from build123d import *

# Parameters (mm, degrees)
F0_W     = 74
F0_H     = 88.5
F1_DEPTH = 34
F2_W     = 70
F2_H     = 83.5
F3_DEPTH = 33
F5_DEPTH = 15
F6_DEPTH = 1
F7_W     = 10
F7_H     = 6
F8_DEPTH = 25


with BuildPart() as f1:
    # F0 (on Top) → F1 (new body)
    with BuildSketch(Plane.XY):
        Rectangle(F0_W, F0_H)
    extrude(amount=F1_DEPTH)

    # F2 (on face) → F3 (cut)
    with BuildSketch(Plane.XY.offset(34)):
        Rectangle(F2_W, F2_H)
    extrude(amount=-F3_DEPTH, mode=Mode.SUBTRACT)

    # F4 (on face) → F5 (join)
    with BuildSketch(Plane.XY.offset(1)):
        with BuildLine():
            ThreePointArc((-7.5, 39.25), (-7.866117, 40.133883), (-8.75, 40.5))
            Line((-8.75, 40.5), (-8.75, 39.25))
            Line((-8.75, 39.25), (-10, 39.25))
            ThreePointArc((-10, 39.25), (-8.75, 38), (-7.5, 39.25))
        make_face()
        with BuildLine():
            Line((-8.75, 39.25), (-8.75, 40.5))
            ThreePointArc((-8.75, 40.5), (-9.633883, 40.133883), (-10, 39.25))
            Line((-10, 39.25), (-8.75, 39.25))
        make_face()
    extrude(amount=F5_DEPTH)

    # F0 (on Top) → F6 (join)
    with BuildSketch(Plane.XY):
        Rectangle(F0_W, F0_H)
    extrude(amount=-F6_DEPTH)

    # F7 (on face) → F8 (cut)
    with BuildSketch(Plane.XZ.offset(44.25)):
        with Locations((-12, 10.5)):
            Rectangle(F7_W, F7_H)
    extrude(amount=-F8_DEPTH, mode=Mode.SUBTRACT)


solid = f1.part
Input: part model. Units: mm. Frame: model coordinates. A direction names the side the tool comes from. Round coordinates to 2 decimals unless told otherwise and drop trailing zeros. Order: outer loops, then holes, each group sorted by start corner. A loop starts at its lowest first (then second) coordinate and runs counter-clockwise, first axis right, second up. Notation, with made-up numbers: (-8, 54) - (49, 54) arc R16 cw to (49, 68) - close; hole circle Ø1 at (2, -35.5). An arc over 180 degrees is marked (long way). Use a Markdown table: item, result.
1. Material intervals for probe 1 along Y at (x, z) = (24.5, 25); probe 2 along X at (y, z) = (-39, 3.5); probe 3 along Y at (x, z) = (-11.5, 12.5), sorted ascending.
Evaluation:
| item | result |
|---|---|
| probe 1 | -44.25 to -41.75, 41.75 to 44.25 |
| probe 2 | -37 to -35, 35 to 37 |
| probe 3 | 41.75 to 44.25 |
2. First-contact query: pin 1 (1.2 mm diameter, centred on x = -9, y = 39, fed in from +Z). Flat tip, straight axial feed; report the tip coordinate or a pass-through.
Evaluation:
| item | result |
|---|---|
| pin 1 | z = 16 |
3. Access query for faces 1 (the face through (0, 1, 1)), 2 (the face through (-12, -43, 7.5)), 3 (the face through (-36, 0, 34)). Directions: +Z, -Z, +X, -X, +Y, -Y. A direction counts if a zero-diameter tool reaches every point of the face in a straight line with its end or side. Return the directions, or none.
Evaluation:
| item | result |
|---|---|
| face 1 | +Z |
| face 2 | -Y |
| face 3 | +Z, +X, -X, +Y, -Y |
4. Section B-B on z = 19. Return the cut outline in (x, y), then the cut area to 3 significant figures.
Evaluation:
| item | result |
|---|---|
| outline | (-37, -44.25) - (37, -44.25) - (37, 44.25) - (-37, 44.25) - close; hole (-35, -41.75) - (35, -41.75) - (35, 41.75) - (-35, 41.75) - close |
| area | 704 mm^2 |
5. Section A-A on z = 3.5. Return the cut outline in (x, y), then the cut area to 3 significant figures.
Evaluation:
| item | result |
|---|---|
| outline | (-37, -44.25) - (37, -44.25) - (37, 44.25) - (-37, 44.25) - close; (-10, 39.25) arc R1.25 ccw to (-7.5, 39.25) arc R1.25 ccw to (-8.75, 40.5) arc R1.25 ccw to start; hole (-35, -41.75) - (35, -41.75) - (35, 41.75) - (-35, 41.75) - close |
| area | 709 mm^2 |
6. Section C-C on y = 20. Return the cut outline in (x, z).
Evaluation:
| item | result |
|---|---|
| outline | (-37, -1) - (37, -1) - (37, 34) - (35, 34) - (35, 1) - (-35, 1) - (-35, 34) - (-37, 34) - close |
7. Section D-D on x = 19. Return the cut outline in (y, z).
Evaluation:
| item | result |
|---|---|
| outline | (-44.25, -1) - (44.25, -1) - (44.25, 34) - (41.75, 34) - (41.75, 1) - (-41.75, 1) - (-41.75, 34) - (-44.25, 34) - close |
8. Mould query, pull axis Z, two halves, no side actions, for faces 4 (the face through (-17, -43, 10)), 5 (the face through (35, -1, 18)), 6 (the face through (-7, -43, 10)), 7 (the face through (-1, 1, -1)). Classes: +Z half, -Z half, draft (parallel to the pull), parting line (faces both ways), or undercut.
Evaluation:
| item | result |
|---|---|
| face 4 | undercut |
| face 5 | draft |
| face 6 | undercut |
| face 7 | -Z half |
